Input: part model. Units: mm. Frame: model coordinates. Round coordinates to 2 decimals unless told otherwise and drop trailing zeros. Loops run counter-clockwise (first coordinate to the right, second up) from the corner with the lowest first, then second, coordinate; pieces in that order, holes last.
1) Draft query along X for faces 1 (the face through (0, 12, 1)), 2 (the face through (44, 12, 1)), 3 (the face through (35, 24, 1)), 4 (the face through (70, 12, 1)). Return one class per face: pulls with the +X half, pulls with the -X half, needs draft (parallel to the pull), parting line crosses it, or undercut.
2) Section C-C, the plane z = 0.6. Return loops of the section in (x, y).
3) Section A-A, the plane y = 10. Return loops of the section in (x, z), and give its area (3 significant figures).
4) Section B-B, the plane x = 36. Return loops of the section in (y, z), and give its area (3 significant figures).
5) Section D-D, the plane x = 43.5. Return loops of the section in (y, z).
6) First-contact query: pin 1 (10 mm diameter, centred on x = 35.5, y = 8, fed in from +Z). Flat tip, straight axial feed; report the tip coordinate or a pass-through.
7) Ray query, line 1 along X through (y, z) = (9, 0.5); line 2 along X through (y, z) = (6, 1.7); line 3 along Y through (x, z) = (25.5, 1.1). Return the intervals inside material, ascending.
Autodesk Inventor part; units mm, degrees
ref_plane "YZ Plane" through (0, 0, 0) normal (1, 0, 0) x (0, 1, 0)
ref_plane "XZ Plane" through (0, 0, 0) normal (0, 1, 0) x (-1, 0, 0)
ref_plane "XY Plane" through (0, 0, 0) normal (0, 0, 1) x (1, 0, 0)
sketch "Sketch1" plane through (0, 0, 0) normal (0, 0, 1) x (1, 0, 0)
  line L0 (0, 0) -> (70, 0)
  line L1 (70, 0) -> (70, 24)
  line L2 (70, 24) -> (0, 24)
  line L3 (0, 24) -> (0, 0)
  line L4 (27.5, 4.5) -> (42.5, 4.5)
  line L5 (42.5, 4.5) -> (42.5, 19.5)
  line L6 (42.5, 19.5) -> (27.5, 19.5)
  line L7 (27.5, 19.5) -> (27.5, 4.5)
  line L8 (27.5, 4.5) -> (42.5, 19.5) construction
  line L9 (42.5, 4.5) -> (27.5, 19.5) construction
  point P0 (35, 12)
  dimension "d0" = 70
  dimension "d1" = 24
  dimension "d2" = 15
  dimension "d3" = 15
extrude "Extrusion1" add sketch "Sketch1" along normal blind 1
sketch "Sketch2" plane through (0, 0, 1) normal (0, 0, 1) x (1, 0, 0)
  line L0 (27.5, 4.5) -> (27.5, 19.5)
  line L1 (27.5, 19.5) -> (42.5, 19.5)
  line L2 (42.5, 19.5) -> (42.5, 4.5)
  line L3 (42.5, 4.5) -> (27.5, 4.5)
  line L4 (0, 0) -> (70, 0)
  line L5 (70, 0) -> (70, 24)
  line L6 (70, 24) -> (0, 24)
  line L7 (0, 24) -> (0, 0)
  line L8 (45, 2) -> (25, 2)
  line L9 (25, 2) -> (25, 22)
  line L10 (25, 22) -> (45, 22)
  line L11 (45, 22) -> (45, 2)
  line L12 (45, 2) -> (25, 22) construction
  line L13 (25, 2) -> (45, 22) construction
  point P0 (35, 12)
  dimension "d6" = 20
  dimension "d7" = 20
extrude "Extrusion2" add sketch "Sketch2" along normal blind 1 contours L7 L6 L5 L4
properties part number "cellSTORM_coverslip_slide_adapter"
Final values:
1. face 1: pulls with the -X half
1. face 2: undercut
1. face 3: needs draft
1. face 4: pulls with the +X half
2. outline: (0, 0) - (70, 0) - (70, 24) - (0, 24) - close; hole (27.5, 4.5) - (42.5, 4.5) - (42.5, 19.5) - (27.5, 19.5) - close
3. outline: (0, 0) - (27.5, 0) - (27.5, 1) - (25, 1) - (25, 2) - (0, 2) - close; (42.5, 0) - (70, 0) - (70, 2) - (45, 2) - (45, 1) - (42.5, 1) - close
3. area: 105 mm2
4. outline: (0, 0) - (4.5, 0) - (4.5, 1) - (2, 1) - (2, 2) - (0, 2) - close; (19.5, 0) - (24, 0) - (24, 2) - (22, 2) - (22, 1) - (19.5, 1) - close
4. area: 13.0 mm2
5. outline: (0, 0) - (24, 0) - (24, 2) - (22, 2) - (22, 1) - (2, 1) - (2, 2) - (0, 2) - close
6. pin 1: stops at z = 1
7. line 1: x = 0 to 27.5, 42.5 to 70
7. line 2: x = 0 to 25, 45 to 70
7. line 3: y = 0 to 2, 22 to 24
